Read the model definition and answer for the solid it produces. Units are mm, in the model's axes. Face numbers are marked on the shaded views. A direction names the side the tool comes from. Round coordinates to 2 decimals unless told otherwise and drop trailing zeros. Write each loop counter-clockwise with the first axis right and the second up, starting at its lowest first coordinate (ties: lowest second). Pieces come first, ordered by that corner, then holes. Notation, with made-up numbers: (-16.75, -5.75) - (22.25, -5.75) arc R26 ccw to (22.25, 24.25) - close; hole circle Ø8 at (2.5, 27.25). An arc over 180 degrees is marked (long way). Answer as CSV lines item,"result". Start each with the question number.
1) Find section A-A on z = -52. Determine the outline of the cut face in (x, y), then the cut area to 3 significant figures.
2) Find section C-C on x = 5.5. Determine the outline of the cut face in (y, z), then the cut area to 3 significant figures.
3) For a pull along Y with two mould halves and no side action, classify the marked faces 3, 4 and 5 as +Y half, -Y half, draft (parallel to the pull), parting line (faces both ways), or undercut.
4) Find section D-D on y = 0. Determine the outline of the cut face in (x, z), then the cut area to 3 significant figures.
5) Find section B-B on y = 7. Determine the outline of the cut face in (x, z), then the cut area to 3 significant figures.
6) Each of these flat-tipped pins is pushed along its axis until it touches: pin 1 (4.5 mm diameter, centred on x = 17.44, z = -14.71, fed in from -Y); pin 2 (6 mm diameter, centred on x = 7, y = -10, fed in from +Z); pin 3 (16.5 mm diameter, centred on x = -2.5, y = 4, fed in from -Z); pin 4 (8.5 mm diameter, centred on x = -20, z = -42.5, fed in from +Y). Where does it stop, or does it pass through?
7) Which of the six approach directions +Z, -Z, +X, -X, +Y, -Y give full straight-line access (tool end or side, diameter ignored) to the marked faces 1 and 2?
8) Consider line 1 along X through (y, z) = (-0.5, -36.5); line 2 along Y through (x, z) = (18, -27); line 3 along Z through (x, y) = (2, -15). Determine where each line is inside the solid, lowest interval first.
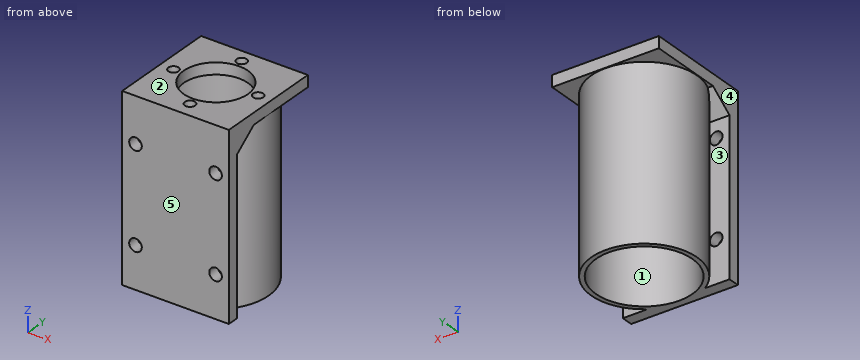
from build123d import *

# Parameters (mm, degrees)
SKETCH1_W           = 46.5
SKETCH1_H           = 46.5
SKETCH1_R           = 14
SKETCH1_R_2         = 2.25
BOSS_EXTRUDE1_DEPTH = 5
SKETCH2_W           = 46.5
SKETCH2_H           = 5
BOSS_EXTRUDE2_DEPTH = 149
SKETCH4_W           = 46.5
SKETCH4_H           = 5
BOSS_EXTRUDE3_DEPTH = 1
SKETCH5_R           = 2.75
CUT_EXTRUDE1_DEPTH  = 10
SKETCH9_R           = 23
CUT_EXTRUDE2_DEPTH  = 149
SKETCH10_R          = 23
SKETCH10_R_2        = 21
BOSS_EXTRUDE4_DEPTH = 149
CHAMFER1_SIZE       = 10
CHAMFER1_SIZE2      = 7.26542528
CHAMFER2_SIZE       = 10
CHAMFER2_SIZE2      = 7.26542528
SKETCH11_W          = 46.5
SKETCH11_H          = 74.694653746
CUT_EXTRUDE3_DEPTH  = 149


with BuildPart() as part:
    # Sketch1 → Boss-Extrude1 (new body)
    with BuildSketch(Plane.XY):
        Rectangle(SKETCH1_W, SKETCH1_H)
        Circle(SKETCH1_R, mode=Mode.SUBTRACT)
        with Locations((-1.381951843, 17.445349211)):
            Circle(SKETCH1_R_2, mode=Mode.SUBTRACT)
        with Locations((17.445349211, 1.381951843)):
            Circle(SKETCH1_R_2, mode=Mode.SUBTRACT)
        with Locations((1.381951843, -17.445349211)):
            Circle(SKETCH1_R_2, mode=Mode.SUBTRACT)
        with Locations((-17.445349211, -1.381951843)):
            Circle(SKETCH1_R_2, mode=Mode.SUBTRACT)
    extrude(amount=BOSS_EXTRUDE1_DEPTH)

    # Sketch2 → Boss-Extrude2 (add)
    with BuildSketch(Plane(origin=(0, 0, 0), x_dir=(-1, 0, 0), z_dir=(0, 0, -1))):
        with Locations((0, -21.75)):
            Rectangle(SKETCH2_W, SKETCH2_H)
    extrude(amount=BOSS_EXTRUDE2_DEPTH)

    # Sketch4 → Boss-Extrude3 (add)
    with BuildSketch(Plane.XZ.offset(23.25)):
        with Locations((0, 2.5)):
            Rectangle(SKETCH4_W, SKETCH4_H)
    extrude(amount=BOSS_EXTRUDE3_DEPTH)

    # Sketch5 → Cut-Extrude1 (cut)
    with BuildSketch(Plane(origin=(0, -19.25, 0), x_dir=(1, 0, 0), z_dir=(0, 1, 0))):
        with Locations((17.443135508, 14.708820521)):
            Circle(SKETCH5_R)
        with Locations((17.443135508, 87.833686256)):
            Circle(SKETCH5_R)
        with Locations((17.443135508, 56.021234434)):
            Circle(SKETCH5_R)
        with Locations((17.443135508, 129.140706858)):
            Circle(SKETCH5_R)
    cut_extrude1 = extrude(amount=-CUT_EXTRUDE1_DEPTH, mode=Mode.SUBTRACT)

    # Mirror1: Cut-Extrude1 across plane
    add(cut_extrude1.mirror(Plane(origin=(0, 0, 0), x_dir=(0, 0, 1), z_dir=(1, 0, 0))), mode=Mode.SUBTRACT)

    # Sketch9 → Cut-Extrude2 (cut)
    with BuildSketch(Plane(origin=(0, 0, -149), x_dir=(-1, 0, 0), z_dir=(0, 0, -1))):
        Circle(SKETCH9_R)
    extrude(amount=-CUT_EXTRUDE2_DEPTH, mode=Mode.SUBTRACT)

    # Sketch10 → Boss-Extrude4 (add)
    with BuildSketch(Plane(origin=(0, 0, -149), x_dir=(-1, 0, 0), z_dir=(0, 0, -1))):
        Circle(SKETCH10_R)
        Circle(SKETCH10_R_2, mode=Mode.SUBTRACT)
    extrude(amount=-BOSS_EXTRUDE4_DEPTH)

    # Chamfer1
    chamfer1_edges = [part.edges().sort_by_distance(p)[0] for p in [
        (17.918597938, -19.25, 0),
    ]]
    chamfer1_side = [part.faces().sort_by_distance(p)[0] for p in [
        (0, 23.062996032, 0),
    ]]
    chamfer(chamfer1_edges, length=CHAMFER1_SIZE, length2=CHAMFER1_SIZE2, reference=chamfer1_side[0])

    # Chamfer2
    chamfer2_edges = [part.edges().sort_by_distance(p)[0] for p in [
        (-17.918597938, -19.25, 0),
    ]]
    chamfer2_side = [part.faces().sort_by_distance(p)[0] for p in [
        (-6.732220056, 22.650656451, 0),
    ]]
    chamfer(chamfer2_edges, length=CHAMFER2_SIZE, length2=CHAMFER2_SIZE2, reference=chamfer2_side[0])

    # Sketch11 → Cut-Extrude3 (cut)
    with BuildSketch(Plane.XZ.offset(24.25)):
        with Locations((0, -111.652673127)):
            Rectangle(SKETCH11_W, SKETCH11_H)
    extrude(amount=-CUT_EXTRUDE3_DEPTH, mode=Mode.SUBTRACT)


solid = part.part
Check values:
1,outline,"(-23.25, -24.25) - (23.25, -24.25) - (23.25, -19.25) - (12.59, -19.25) arc R23 ccw (long way) to (-12.59, -19.25) - (-23.25, -19.25) - close; hole circle Ø42 at (0, 0)"
1,area,"445 mm^2"
2,outline,"(-24.25, -74.31) - (-20.27, -74.31) - (-20.27, 0) - (-12.87, 0) - (-12.87, 5) - (-24.25, 5) - close; (12.87, 0) - (20.27, 0) - (20.27, -74.31) - (22.33, -74.31) - (22.33, 0) - (23.25, 0) - (23.25, 5) - (12.87, 5) - close"
2,area,"558 mm^2"
3,face 3,"undercut"
3,face 4,"draft"
3,face 5,"-Y half"
4,outline,"(-23.25, 0) - (-23, 0) - (-23, -74.31) - (-21, -74.31) - (-21, 0) - (-19.22, 0) - (-19.22, 5) - (-23.25, 5) - close; (-15.67, 0) - (-14, 0) - (-14, 5) - (-15.67, 5) - close; (14, 0) - (15.67, 0) - (15.67, 5) - (14, 5) - close; (19.22, 0) - (21, 0) - (21, -74.31) - (23, -74.31) - (23, 0) - (23.25, 0) - (23.25, 5) - (19.22, 5) - close"
4,area,"354 mm^2"
5,outline,"(-23.25, 0) - (-21.91, 0) - (-21.91, -74.31) - (-19.8, -74.31) - (-19.8, 0) - (-12.12, 0) - (-12.12, 5) - (-23.25, 5) - close; (12.12, 0) - (19.8, 0) - (19.8, -74.31) - (21.91, -74.31) - (21.91, 0) - (23.25, 0) - (23.25, 5) - (12.12, 5) - close"
5,area,"425 mm^2"
6,pin 1,"stops at y = -17.27"
6,pin 2,"stops at z = 5"
6,pin 3,"passes through"
6,pin 4,"stops at y = 16.76"
7,face 1,"-Z"
7,face 2,"+Z, +X, -X, +Y, -Y"
8,line 1,"x = -22.99 to -20.99, 20.99 to 22.99"
8,line 2,"y = -24.25 to -19.25, -14.32 to -10.82, 10.82 to 14.32"
8,line 3,"z = 0 to 5"
